Can you work these out from the model? Positions are in its coordinate system, mm. A direction names the side the tool comes from. Give positions to 0.01 mm unless a question says otherwise; leave off trailing zeros. Loops run counter-clockwise (first coordinate to the right, second up) from the corner with the lowest first, then second, coordinate; pieces in that order, holes last.
from build123d import *

# Parameters (mm, degrees)
SKETCH_1_W           = 250
SKETCH_1_H           = 150
EXTRUDE_1_DEPTH      = 1.5
SKETCH_2_W           = 40
SKETCH_2_H           = 50
CUT_EXTRUDE_1_DEPTH  = 233.650381036
SKETCH_3_W           = 40
SKETCH_3_H           = 50
CUT_EXTRUDE_2_DEPTH  = 233.650381036
CUT_EXTRUDE_3_DEPTH  = 233.650381036
SKETCH_5_W           = 100
SKETCH_5_H           = 10
CUT_EXTRUDE_4_DEPTH  = 233.650381036
EXTRUDE_2_DEPTH      = 100
EXTRUDE_3_DEPTH      = 100
CUT_EXTRUDE_5_DEPTH  = 268.016260599
CUT_EXTRUDE_7_DEPTH  = 10
SKETCH_14_W          = 50
SKETCH_14_H          = 58.309518949
CUT_EXTRUDE_10_DEPTH = 10
SKETCH_15_R          = 16
CUT_EXTRUDE_11_DEPTH = 10
CUT_EXTRUDE_14_DEPTH = 268.016260599
SKETCH_20_W          = 40
SKETCH_20_H          = 50
CUT_EXTRUDE_15_DEPTH = 10
FILLET_1_R           = 3
SKETCH_21_W          = 2
SKETCH_21_H          = 30
CUT_EXTRUDE_16_DEPTH = 10


with BuildPart() as part:
    # 草图1 → 凸台-拉伸1 (new body)
    with BuildSketch(Plane.XY):
        with Locations((71.202531646, -50.014064698)):
            Rectangle(SKETCH_1_W, SKETCH_1_H)
    extrude(amount=EXTRUDE_1_DEPTH)

    # 草图2 → 切除-拉伸1 (cut, through all)
    with BuildSketch(Plane.XY.offset(1.5)):
        with Locations((-33.797468354, -0.014064698)):
            Rectangle(SKETCH_2_W, SKETCH_2_H)
    extrude(amount=-CUT_EXTRUDE_1_DEPTH, mode=Mode.SUBTRACT)

    # 草图3 → 切除-拉伸2 (cut, through all)
    with BuildSketch(Plane.XY.offset(1.5)):
        with Locations((-33.797468354, -100.014064698)):
            Rectangle(SKETCH_3_W, SKETCH_3_H)
    extrude(amount=-CUT_EXTRUDE_2_DEPTH, mode=Mode.SUBTRACT)

    # 草图4 → 切除-拉伸3 (cut, through all)
    with BuildSketch(Plane.XY.offset(1.5)):
        Polygon((-13.797468354, -75.014064698), (16.202531646, -125.014064698), (-13.797468354, -125.014064698), align=None)
        Polygon((-13.797468354, -25.014064698), (16.202531646, 24.985935302), (-13.797468354, 24.985935302), align=None)
    extrude(amount=-CUT_EXTRUDE_3_DEPTH, mode=Mode.SUBTRACT)

    # 草图5 → 切除-拉伸4 (cut, through all)
    with BuildSketch(Plane.XY.offset(1.5)):
        with Locations((96.202531646, -60.014064698)):
            Rectangle(SKETCH_5_W, SKETCH_5_H)
        with Locations((96.202531646, -40.014064698)):
            Rectangle(SKETCH_5_W, SKETCH_5_H)
    extrude(amount=-CUT_EXTRUDE_4_DEPTH, mode=Mode.SUBTRACT)

    # 草图6 → 凸台-拉伸2 (add)
    with BuildSketch(Plane.XY.offset(1.5)):
        Polygon((-13.797468354, -75.014064698), (-9.06108927, -75.014064698), (17.975201528, -120.010528641), (191.672994216, -120.010528641), (191.672994216, 24.985935302), (196.202531646, 24.985935302), (196.202531646, -125.014064698), (16.202531646, -125.014064698), align=None)
    extrude(amount=EXTRUDE_2_DEPTH)

    # 草图7 → 凸台-拉伸3 (add)
    with BuildSketch(Plane.XY.offset(1.5)):
        Polygon((-9.70187004, -26.373391519), (17.639126857, 19.845802477), (191.672994216, 19.845802477), (191.672994216, 24.985935302), (16.202531646, 24.985935302), (-13.797468354, -25.014064698), align=None)
    extrude(amount=EXTRUDE_3_DEPTH)

    # 草图8 → 切除-拉伸5 (cut, through all)
    with BuildSketch(Plane(origin=(0, 24.985935302, 0), x_dir=(1, 0, 0), z_dir=(0, 1, 0))):
        Polygon((179.466999768, -10.18289615), (165.324864144, -24.325031774), (165.324864144, -19.325031774), (179.466999768, -5.18289615), align=None)
        Polygon((163.399705406, -10.407679967), (149.257569782, -24.549815591), (149.257569782, -19.549815591), (163.399705406, -5.407679967), align=None)
        Polygon((124.257569782, -24.549815591), (124.257569782, -19.549815591), (138.399705406, -5.407679967), (138.399705406, -10.407679967), align=None)
        Polygon((99.257569782, -24.549815591), (99.257569782, -19.549815591), (113.399705406, -5.407679967), (113.399705406, -10.407679967), align=None)
        Polygon((74.257569782, -24.549815591), (74.257569782, -19.549815591), (88.399705406, -5.407679967), (88.399705406, -10.407679967), align=None)
        Polygon((49.257569782, -24.549815591), (49.257569782, -19.549815591), (63.399705406, -5.407679967), (63.399705406, -10.407679967), align=None)
        Polygon((24.257569782, -24.549815591), (24.257569782, -19.549815591), (38.399705406, -5.407679967), (38.399705406, -10.407679967), align=None)
    extrude(amount=-CUT_EXTRUDE_5_DEPTH, mode=Mode.SUBTRACT)

    # 草图11 → 切除-拉伸7 (cut)
    with BuildSketch(Plane(origin=(-43.239637627, -25.943782576, 0), x_dir=(0, 0, 1), z_dir=(-0.8574929257125441, -0.5144957554275268, 0))):
        Polygon((101.5, -57.225290903), (51.5, -57.225290903), (50.75, -115.534809852), (101.5, -115.534809852), align=None)
    extrude(amount=-CUT_EXTRUDE_7_DEPTH, mode=Mode.SUBTRACT)

    # 草图14 → 切除-拉伸10 (cut)
    with BuildSketch(Plane(origin=(0.890419459, -0.534251675, 0), x_dir=(0, 0, 1), z_dir=(-0.8574929257125442, 0.5144957554275266, 0))):
        with Locations((76.5, 0.606637048)):
            Rectangle(SKETCH_14_W, SKETCH_14_H)
    extrude(amount=-CUT_EXTRUDE_10_DEPTH, mode=Mode.SUBTRACT)

    # 草图15 → 切除-拉伸11 (cut)
    with BuildSketch(Plane(origin=(-43.239637627, -25.943782576, 0), x_dir=(0, 0, 1), z_dir=(-0.8574929257125441, -0.5144957554275268, 0))):
        with Locations(Location((26.124922648, -86.225290903, 0), (0, 0, 270))):
            Circle(SKETCH_15_R)
    extrude(amount=-CUT_EXTRUDE_11_DEPTH, mode=Mode.SUBTRACT)

    # 草图19 → 切除-拉伸14 (cut, through all)
    with BuildSketch(Plane(origin=(0, 24.985935302, 0), x_dir=(1, 0, 0), z_dir=(0, 1, 0))):
        Polygon((46.202531646, -101.5), (16.202531646, -51.5), (16.202531646, -101.5), align=None)
    extrude(amount=-CUT_EXTRUDE_14_DEPTH, mode=Mode.SUBTRACT)

    # 草图20 → 切除-拉伸15 (cut)
    with BuildSketch(Plane(origin=(196.202531646, 0, 0), x_dir=(0, 0, -1), z_dir=(1, 0, 0))):
        with Locations((-51.207849099, -50.014064698)):
            Rectangle(SKETCH_20_W, SKETCH_20_H)
    extrude(amount=-CUT_EXTRUDE_15_DEPTH, mode=Mode.SUBTRACT)

    # 圆角1
    fillet_1_edges = [part.edges().sort_by_distance(p)[0] for p in [
        (106.202531646, -125.014064698, 0),
        (106.202531646, 24.985935302, 0),
        (196.202531646, -50.014064698, 0),
        (196.202531646, 24.985935302, 50.75),
        (196.202531646, -125.014064698, 50.75),
    ]]
    fillet(fillet_1_edges, radius=FILLET_1_R)

    # 草图21 → 切除-拉伸16 (cut)
    with BuildSketch(Plane(origin=(196.202531646, 0, 0), x_dir=(0, 0, -1), z_dir=(1, 0, 0))):
        with Locations((-63.800605611, -97.014064698)):
            Rectangle(SKETCH_21_W, SKETCH_21_H)
        with Locations((-73.750757013, -97.014064698)):
            Rectangle(SKETCH_21_W, SKETCH_21_H)
        with Locations((-53.850454208, -97.014064698)):
            Rectangle(SKETCH_21_W, SKETCH_21_H)
        with Locations((-43.900302805, -97.014064698)):
            Rectangle(SKETCH_21_W, SKETCH_21_H)
        with Locations((-33.950151403, -97.014064698)):
            Rectangle(SKETCH_21_W, SKETCH_21_H)
        with Locations((-24, -97.014064698)):
            Rectangle(SKETCH_21_W, SKETCH_21_H)
        with Locations((-64.626123933, -3.300353784)):
            Rectangle(SKETCH_21_W, SKETCH_21_H)
        with Locations((-74.626123933, -3.300353784)):
            Rectangle(SKETCH_21_W, SKETCH_21_H)
        with Locations((-54.626123933, -3.300353784)):
            Rectangle(SKETCH_21_W, SKETCH_21_H)
        with Locations((-44.626123933, -3.300353784)):
            Rectangle(SKETCH_21_W, SKETCH_21_H)
        with Locations((-34.626123933, -3.300353784)):
            Rectangle(SKETCH_21_W, SKETCH_21_H)
        with Locations((-24, -3.014064698)):
            Rectangle(SKETCH_21_W, SKETCH_21_H)
    extrude(amount=-CUT_EXTRUDE_16_DEPTH, mode=Mode.SUBTRACT)


solid = part.part
(1) Suppose I cut it at D-D on z = 88. List the corners of the cut face in (x, y) for me, plus the area to 3 significant figures.
Returned:
outline: (38.1, -125.01) - (193.2, -125.01) arc R3 ccw to (196.2, -122.01) - (196.2, 21.99) arc R3 ccw to (193.2, 24.99) - (38.1, 24.99) - (38.1, 19.85) - (191.67, 19.85) - (191.67, -120.01) - (38.1, -120.01) - close
area: 2,230 mm2
(2) Suppose I cut it at A-A on x = 95.5. List the corners of the cut face in (y, z) for me, plus the area to 3 significant figures.
Returned:
outline: (-125.01, 3) arc R3 ccw to (-122.01, 0) - (-65.01, 0) - (-65.01, 1.5) - (-120.01, 1.5) - (-120.01, 101.5) - (-125.01, 101.5) - close; (-55.01, 0) - (-45.01, 0) - (-45.01, 1.5) - (-55.01, 1.5) - close; (-35.01, 0) - (21.99, 0) arc R3 ccw to (24.99, 3) - (24.99, 101.5) - (19.85, 101.5) - (19.85, 1.5) - (-35.01, 1.5) - close
area: 1,210 mm2
(3) Thinking about a two-plate mould opening in Y: for faces 4 (the cylindrical face through (7.277, -106.22, 39.616)), 5 (the flat face through (56.43, -122.48, 17.38)), which applies, pulls with the +Y half, pulls with the -Y half, needs draft (parallel to the pull), parting line crosses it, or undercut?
Returned:
face 4: undercut
face 5: needs draft
(4) Please list where these lines run through material, in increasing order: probe 1 along Y at (x, z) = (142.5, 11.5); probe 2 along Z at (x, y) = (74, -79.5); probe 3 along X at (y, z) = (-93, 50).
Returned:
probe 1: y = -125.01 to -120.01, 19.85 to 24.99
probe 2: z = 0 to 1.5
probe 3: x = -3.01 to 1.75, 191.67 to 196.2
(5) Which directions (+Z, -Z, +X, -X, +Y, -Y) give clear straight access to the entire face, cutting with the end or side of a thin tool? Please do faces 1 (the flat face through (-1.74, -87.2, 15.03)), 2 (the flat face through (156.43, 22.45, 17.38)), 3 (the flat face through (-11, -75.014, 26)).
Returned:
face 1: +Z
face 2: +Y, -Y
face 3: +Z, -X
(6) Suppose I cut it at B-B on y = -7. Give the number of separate pieces and of enclosed holes in the cut face, plus the area to 3 significant figures.
Returned:
separate pieces: 7
enclosed holes: 0
area: 933 mm2
(7) Will these pins go through, and if not, where does the flat tip stop? P1, Ø2.5, axis at y = 22.5, z = 7, coming from the -X side; P2, Ø1.4, axis at x = 194.5, z = 46.5, coming from the -Y side; P3, Ø1.6, axis at x = -31, z = 0.5, coming from the -Y side; P4, Ø5.5, axis at y = 23, z = 22.5, coming from the +X side.
Returned:
P1: stops at x = 13.96
P2: stops at y = -124.95
P3: stops at y = -75.01
P4: stops at x = 196.2
